Geometry check sheet. Reference: the model listing, model coordinates, mm. A direction names the side the tool comes from. Give positions to 0.01 mm unless a question says otherwise; leave off trailing zeros. Write each loop counter-clockwise with the first axis right and the second up, starting at its lowest first coordinate (ties: lowest second). Pieces come first, ordered by that corner, then holes. Notation, with made-up numbers: (-1, 23.5) -> (53, 23.5) arc R32 ccw to (53, 55.5) -> close; hole circle Ø11 at (-12, -0.5). An arc over 180 degrees is marked (long way). Write item = value, one per line. Start each with the question number.
1. Cross-section at A-A, the plane x = 7.5. Record the cut outline in (y, z) (3 decimals).
2. Cross-section at D-D, the plane x = 0. Record the cut outline in (y, z) (3 decimals).
3. Set-up check for faces 1 (the flat face through (0, 18.785, 1)), 2 (the flat face through (-12.435, 0, 2)): record each of +Z, -Z, +X, -X, +Y, -Y from which the full face is reachable in a straight line by a thin tool's end or side.
4. Cross-section at C-C, the plane y = -1.5. Record the cut outline in (x, z) (3 decimals), plus the area to 3 significant figures.
5. Thickness scan on line 1 along Y through (x, z) = (4, 1.2) (3 decimals); line 2 along X through (y, z) = (-4, 1.35) (3 decimals); line 3 along X through (y, z) = (13.5, 1.8) (3 decimals). Record the ranges inside material, lowest first.
6. Mould release check, pull along Y, two halves, no side actions. Record for faces 3 (the flat face through (0, -18.785, 1)), 4 (the flat face through (-15.435, 0, 2)), 5 (the flat face through (0, 0, 0)): pulls with the +Y half, pulls with the -Y half, needs draft (parallel to the pull), parting line crosses it, or undercut.
7. Cross-section at B-B, the plane z = 1.45. Record the cut outline in (x, y) (3 decimals), plus the area to 3 significant figures.
```python
from build123d import *

# Parameters (mm, degrees)
SKETCH1_W                 = 37.57
SKETCH1_H                 = 37.57
SKETCH1_W_2               = 3
SKETCH1_H_2               = 3
SKETCH1_H_3               = 5
PLATE_THICKNESS_3MM_DEPTH = 3
SKETCH_1_W                = 3
SKETCH_1_H                = 0.35
SKETCH_1_W_2              = 0.35
SKETCH_1_H_2              = 3.026917622
SKETCH_1_H_3              = 3
CUT_EXTRUDE_1_DEPTH       = 3
SKETCH_1_2_W              = 0.35
SKETCH_1_2_H              = 3
SKETCH_1_2_W_2            = 3
SKETCH_1_2_H_2            = 0.35
EXTRUDE_1_DEPTH           = 3
SKETCH_2_W                = 3
SKETCH_2_H                = 3.5
SKETCH_2_H_2              = 2.5
SKETCH_2_W_2              = 3.5
SKETCH_2_H_3              = 3
CUT_EXTRUDE_2_DEPTH       = 3


with BuildPart() as part:
    # Sketch1 → Plate_thickness_3mm (new body)
    with BuildSketch(Plane.XY):
        Rectangle(SKETCH1_W, SKETCH1_H)
        with Locations((0, -14.285)):
            Rectangle(SKETCH1_W_2, SKETCH1_H_2, mode=Mode.SUBTRACT)
        with Locations((14.285, 0)):
            Rectangle(SKETCH1_W_2, SKETCH1_H_2, mode=Mode.SUBTRACT)
        with Locations((-14.285, 0)):
            Rectangle(SKETCH1_W_2, SKETCH1_H_2, mode=Mode.SUBTRACT)
        with Locations((-8.25, 0)):
            Rectangle(SKETCH1_W_2, SKETCH1_H_3, mode=Mode.SUBTRACT)
        with Locations((0, 14.285)):
            Rectangle(SKETCH1_W_2, SKETCH1_H_2, mode=Mode.SUBTRACT)
        with Locations((8.25, 0)):
            Rectangle(SKETCH1_W_2, SKETCH1_H_3, mode=Mode.SUBTRACT)
    extrude(amount=PLATE_THICKNESS_3MM_DEPTH)

    # 草图1 → 切除-拉伸1 (cut)
    with BuildSketch(Plane.XY.offset(3)):
        with Locations((0, 12.61)):
            Rectangle(SKETCH_1_W, SKETCH_1_H)
        with Locations((-12.61, -0.013458811)):
            Rectangle(SKETCH_1_W_2, SKETCH_1_H_2)
        with Locations((12.61, -0.013458811)):
            Rectangle(SKETCH_1_W_2, SKETCH_1_H_2)
        with Locations((0, -12.61)):
            Rectangle(SKETCH_1_W, SKETCH_1_H)
        with Locations((-15.61, 0)):
            Rectangle(SKETCH_1_W_2, SKETCH_1_H_3)
        with Locations((0, 15.61)):
            Rectangle(SKETCH_1_W, SKETCH_1_H)
        with Locations((15.61, 0)):
            Rectangle(SKETCH_1_W_2, SKETCH_1_H_3)
        with Locations((0, -15.61)):
            Rectangle(SKETCH_1_W, SKETCH_1_H)
    extrude(amount=-CUT_EXTRUDE_1_DEPTH, mode=Mode.SUBTRACT)

    # 草图1<2> → 凸台-拉伸1 (add)
    with BuildSketch(Plane.XY.offset(3)):
        with Locations((-15.61, 0)):
            Rectangle(SKETCH_1_2_W, SKETCH_1_2_H)
        with Locations((0, 15.61)):
            Rectangle(SKETCH_1_2_W_2, SKETCH_1_2_H_2)
        with Locations((15.61, 0)):
            Rectangle(SKETCH_1_2_W, SKETCH_1_2_H)
        with Locations((0, -15.61)):
            Rectangle(SKETCH_1_2_W_2, SKETCH_1_2_H_2)
    extrude(amount=-EXTRUDE_1_DEPTH)

    # 草图2 → 切除-拉伸2 (cut)
    with BuildSketch(Plane.XY.offset(3)):
        with Locations((-13.935, 3.25)):
            Rectangle(SKETCH_2_W, SKETCH_2_H)
        with Locations((-8.25, 3.75)):
            Rectangle(SKETCH_2_W, SKETCH_2_H_2)
        with Locations((-8.25, -3.75)):
            Rectangle(SKETCH_2_W, SKETCH_2_H_2)
        Polygon((-12.785, -1.5), (-15.435, -1.5), (-15.435, -5), (-12.435, -5), (-12.435, -1.526917622), (-12.785, -1.526917622), align=None)
        with Locations((-3.25, 13.935)):
            Rectangle(SKETCH_2_W_2, SKETCH_2_H_3)
        with Locations((3.25, 13.935)):
            Rectangle(SKETCH_2_W_2, SKETCH_2_H_3)
        with Locations((8.25, 3.75)):
            Rectangle(SKETCH_2_W, SKETCH_2_H_2)
        with Locations((13.935, 3.25)):
            Rectangle(SKETCH_2_W, SKETCH_2_H)
        Polygon((12.785, -1.526917622), (12.435, -1.526917622), (12.435, -5), (15.435, -5), (15.435, -1.5), (12.785, -1.5), align=None)
        with Locations((8.25, -3.75)):
            Rectangle(SKETCH_2_W, SKETCH_2_H_2)
        with Locations((3.25, -13.935)):
            Rectangle(SKETCH_2_W_2, SKETCH_2_H_3)
        with Locations((-3.25, -13.935)):
            Rectangle(SKETCH_2_W_2, SKETCH_2_H_3)
    extrude(amount=-CUT_EXTRUDE_2_DEPTH, mode=Mode.SUBTRACT)


solid = part.part
```
Answers:
q1.outline = (-18.785, 0) -> (-5, 0) -> (-5, 3) -> (-18.785, 3) -> close; (5, 0) -> (18.785, 0) -> (18.785, 3) -> (5, 3) -> close
q2.outline = (-18.785, 0) -> (-15.435, 0) -> (-15.435, 3) -> (-18.785, 3) -> close; (-12.435, 0) -> (12.435, 0) -> (12.435, 3) -> (-12.435, 3) -> close; (15.435, 0) -> (18.785, 0) -> (18.785, 3) -> (15.435, 3) -> close
q3.face_1 = +Z, -Z, +X, -X, +Y
q3.face_2 = +Z, -Z
q4.outline = (-18.785, 0) -> (-15.435, 0) -> (-15.435, 3) -> (-18.785, 3) -> close; (-12.435, 0) -> (-9.75, 0) -> (-9.75, 3) -> (-12.435, 3) -> close; (-6.75, 0) -> (6.75, 0) -> (6.75, 3) -> (-6.75, 3) -> close; (9.75, 0) -> (12.435, 0) -> (12.435, 3) -> (9.75, 3) -> close; (15.435, 0) -> (18.785, 0) -> (18.785, 3) -> (15.435, 3) -> close
q4.area = 76.7 mm^2
q5.line_1 = -18.785 to -15.435, -12.435 to 12.435, 15.435 to 18.785
q5.line_2 = -18.785 to -15.435, -12.435 to -9.75, -6.75 to 6.75, 9.75 to 12.435, 15.435 to 18.785
q5.line_3 = -18.785 to -5, 5 to 18.785
q6.face_3 = pulls with the -Y half
q6.face_4 = undercut
q6.face_5 = needs draft
q7.outline = (-18.785, -18.785) -> (18.785, -18.785) -> (18.785, 18.785) -> (-18.785, 18.785) -> close; hole (-15.435, -5) -> (-12.435, -5) -> (-12.435, 5) -> (-15.435, 5) -> close; hole (-9.75, -5) -> (-6.75, -5) -> (-6.75, 5) -> (-9.75, 5) -> close; hole (-5, -15.435) -> (5, -15.435) -> (5, -12.435) -> (-5, -12.435) -> close; hole (-5, 12.435) -> (5, 12.435) -> (5, 15.435) -> (-5, 15.435) -> close; hole (6.75, -5) -> (9.75, -5) -> (9.75, 5) -> (6.75, 5) -> close; hole (12.435, -5) -> (15.435, -5) -> (15.435, 5) -> (12.435, 5) -> close
q7.area = 1,230 mm^2
